Geometry check sheet. Reference: drawing and pictorial views, mm from the part's lowest x, y, z. Round coordinates to 2 decimals unless told otherwise and drop trailing zeros. Write each loop counter-clockwise with the first axis right and the second up, starting at its lowest first coordinate (ties: lowest second). Pieces come first, ordered by that corner, then holes. Notation, with made-up numbers: M 45,-21 L 63,-21 A34 ccw 63,14 Z; hole C 54,-17 d5. An arc over 180 degrees is marked long. One line per question, with ' | ' between items.
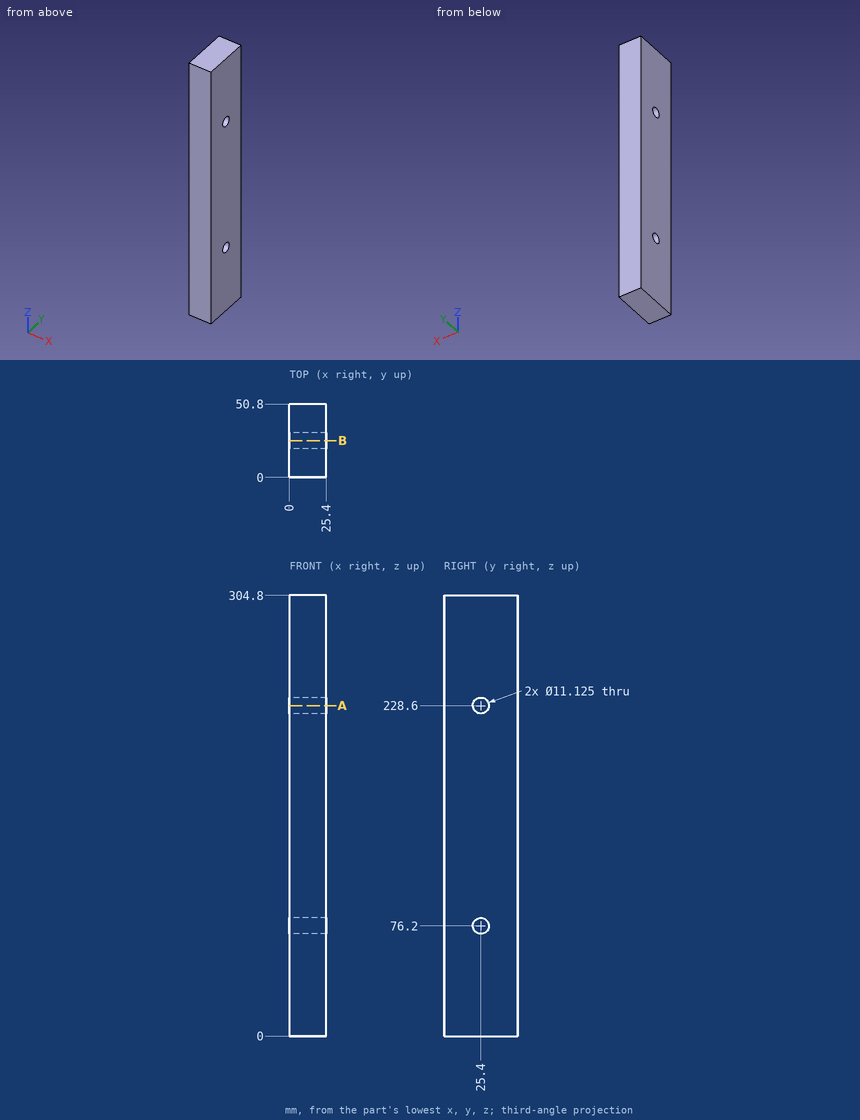
1. Section check B-B, the plane y = 25.4. Record the cut outline in (x, z), then the cut area to 3 significant figures.
Results:
outline: M 0,0 L 25.4,0 L 25.4,70.64 L 0,70.64 Z; M 0,81.76 L 25.4,81.76 L 25.4,223.04 L 0,223.04 Z; M 0,234.16 L 25.4,234.16 L 25.4,304.8 L 0,304.8 Z | area: 7,180 mm2
2. Section check A-A, the plane z = 228.6. Record the cut outline in (x, y), then the cut area to 3 significant figures.
Results:
outline: M 0,0 L 25.4,0 L 25.4,19.84 L 0,19.84 Z; M 0,30.96 L 25.4,30.96 L 25.4,50.8 L 0,50.8 Z | area: 1,010 mm2
3. Thickness scan on line 1 (Z direction, x = 8.75, y = 25.4); line 2 (Y direction, x = 9, z = 76.2). Record the ranges inside material, lowest first.
Results:
line 1: z = 0 to 70.64, 81.76 to 223.04, 234.16 to 304.8 | line 2: y = 0 to 19.84, 30.96 to 50.8
